Answer from the drawing. Dimensions are ordinates in mm from the lowest x, y and z of the part. A direction names the side the tool comes from. Coordinates: 2 decimals unless noted, no trailing zeros. Order: outer loops, then holes, each group sorted by start corner. A loop starts at its lowest first (then second) coordinate and runs counter-clockwise, first axis right, second up. Notation, with made-up numbers: (51.25, 4.5) -> (67.25, 4.5) arc R14 cw to (67.25, 8.5) -> close; hole circle Ø2 at (-17.5, 11.5). An arc over 180 degrees is marked (long way). Answer in a Markdown table with one row per item.
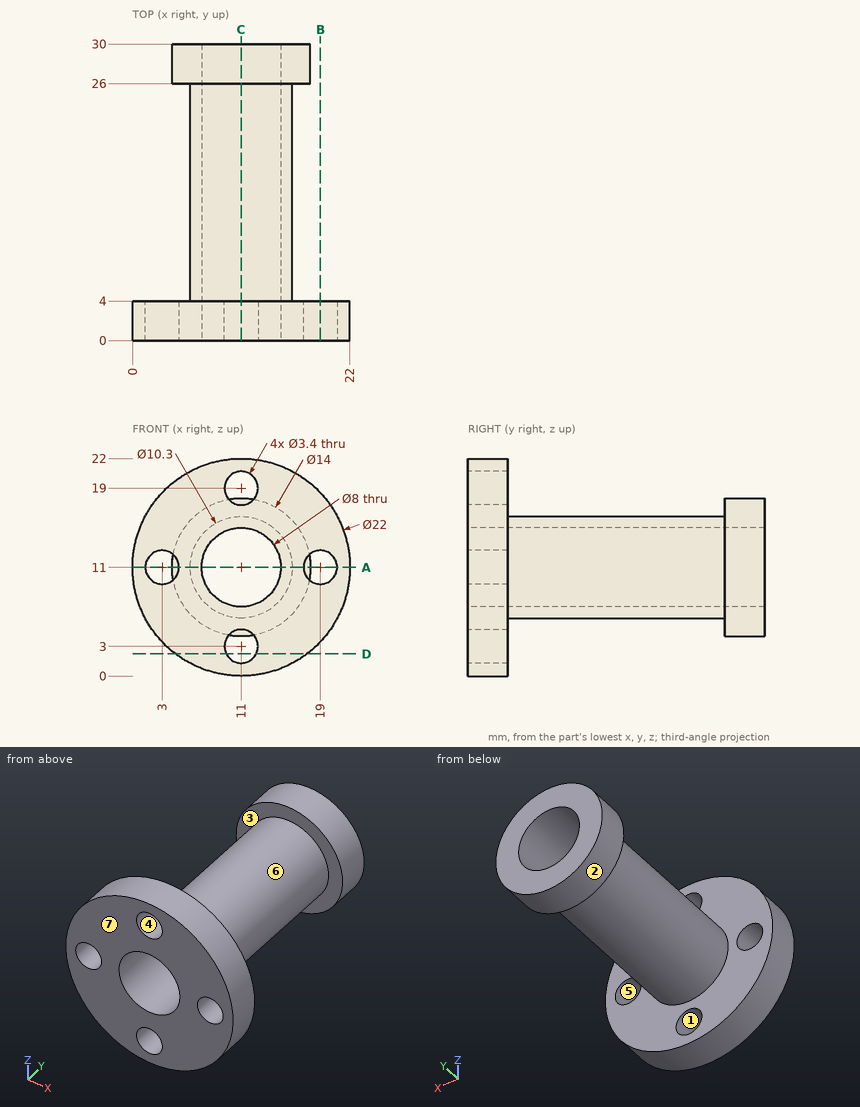
(1) A cutting plane is placed at D-D, the plane z = 2.25. Determine the outline of the cut face in (x, y), then the cut area to 3 significant figures.
Check values:
| item | result |
|---|---|
| outline | (4.33, 0) -> (9.47, 0) -> (9.47, 4) -> (4.33, 4) -> close; (12.53, 0) -> (17.67, 0) -> (17.67, 4) -> (12.53, 4) -> close |
| area | 41.1 mm² |
(2) Flat-ended cylindrical pins translate along their axes: pin 1 (12 mm diameter, centred on x = 17.5, y = 5, fed in from +Z); pin 2 (10 mm diameter, centred on x = 10, z = 12, fed in from -Y); pin 3 (6 mm diameter, centred on x = 9, y = 14.5, fed in from -Z); pin 4 (8 mm diameter, centred on x = 14.5, y = 23, fed in from +Z). Find the tip coordinate at first contact, or state that the pin passes through.
Check values:
| item | result |
|---|---|
| pin 1 | z = 21.98 |
| pin 2 | y = 0 |
| pin 3 | z = 5.85 |
| pin 4 | z = 17.95 |
(3) A cutting plane is placed at B-B, the plane x = 19. Determine the outline of the cut face in (y, z).
Check values:
| item | result |
|---|---|
| outline | (0, 3.45) -> (4, 3.45) -> (4, 9.3) -> (0, 9.3) -> close; (0, 12.7) -> (4, 12.7) -> (4, 18.55) -> (0, 18.55) -> close |
(4) Which of the six approach directions +Z, -Z, +X, -X, +Y, -Y give full straight-line access (tool end or side, diameter ignored) to the marked faces 5, 6 and 7?
Check values:
| item | result |
|---|---|
| face 5 | -Y |
| face 6 | none |
| face 7 | +Z, -Z, +X, -X, -Y |
(5) For a pull along Z with two mould halves and no side action, classify the marked faces 1, 2, 3 and 4 as released by +Z, released by -Z, zero draft, split by the parting line, or undercut.
Check values:
| item | result |
|---|---|
| face 1 | undercut |
| face 2 | split by the parting line |
| face 3 | zero draft |
| face 4 | undercut |
(6) Find the intervals of material crossed by line 1 along X through (y, z) = (1.65, 11); line 2 along Z through (x, y) = (11, 18); line 3 along Y through (x, z) = (5.75, 9.75), in increasing order. Write a range as from..to.
Check values:
| item | result |
|---|---|
| line 1 | 0..1.3, 4.7..7, 15..17.3, 20.7..22 |
| line 2 | 5.85..7, 15..16.15 |
| line 3 | 0..4, 26..30 |
(7) A cutting plane is placed at C-C, the plane x = 11. Determine the outline of the cut face in (y, z), then the cut area to 3 significant figures.
Check values:
| item | result |
|---|---|
| outline | (0, 0) -> (4, 0) -> (4, 1.3) -> (0, 1.3) -> close; (0, 4.7) -> (4, 4.7) -> (4, 5.85) -> (26, 5.85) -> (26, 4) -> (30, 4) -> (30, 7) -> (0, 7) -> close; (0, 15) -> (30, 15) -> (30, 18) -> (26, 18) -> (26, 16.15) -> (4, 16.15) -> (4, 17.3) -> (0, 17.3) -> close; (0, 20.7) -> (4, 20.7) -> (4, 22) -> (0, 22) -> close |
| area | 103 mm² |
(8) A cutting plane is placed at A-A, the plane z = 11. Determine the outline of the cut face in (x, y).
Check values:
| item | result |
|---|---|
| outline | (0, 0) -> (1.3, 0) -> (1.3, 4) -> (0, 4) -> close; (4, 26) -> (5.85, 26) -> (5.85, 4) -> (4.7, 4) -> (4.7, 0) -> (7, 0) -> (7, 30) -> (4, 30) -> close; (15, 0) -> (17.3, 0) -> (17.3, 4) -> (16.15, 4) -> (16.15, 26) -> (18, 26) -> (18, 30) -> (15, 30) -> close; (20.7, 0) -> (22, 0) -> (22, 4) -> (20.7, 4) -> close |
